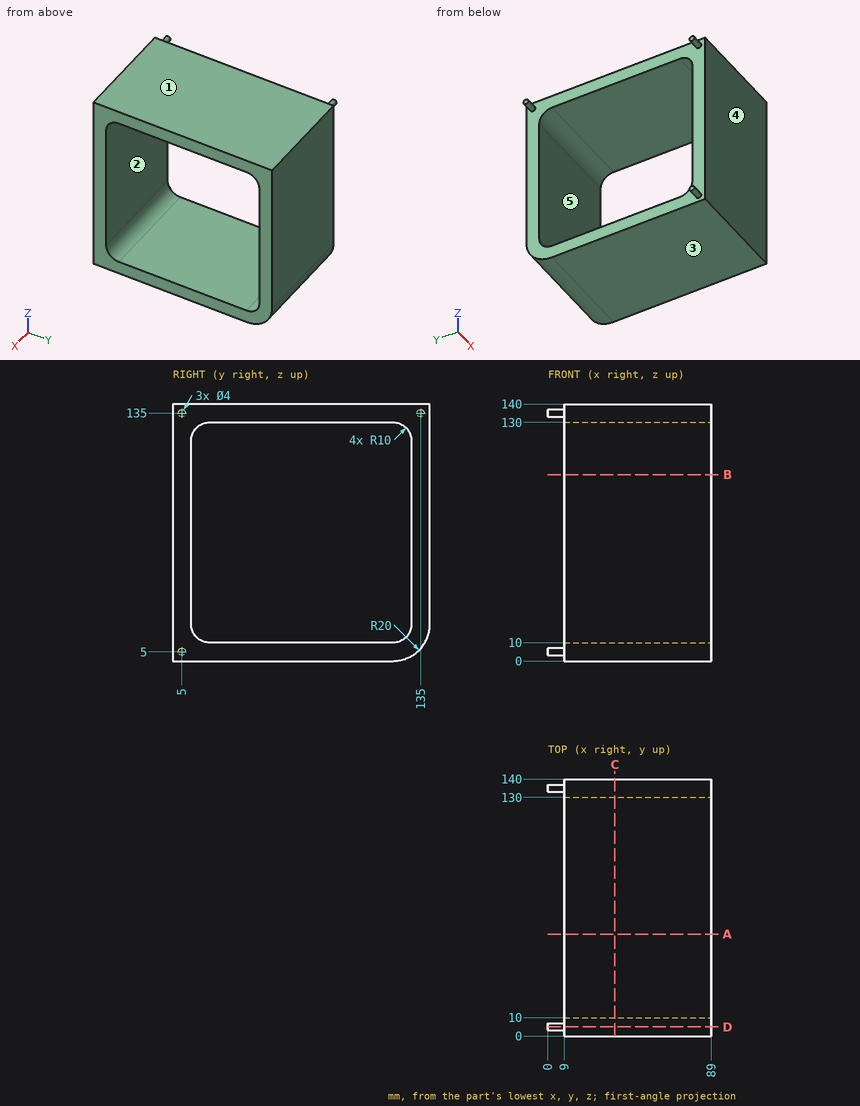
Input: dimensioned drawing with shaded views. Units: mm. Origin: part minimum x, y, z. A direction names the side the tool comes from. Coordinates: 2 decimals unless noted, no trailing zeros. Write each loop counter-clockwise with the first axis right and the second up, starting at its lowest first coordinate (ties: lowest second). Pieces come first, ordered by that corner, then holes. Notation, with made-up numbers: M -39.5,53.25 L -8.5,53.25 A16 cw -8.5,74.25 Z; hole C 41.5,84.25 d1. An arc over 180 degrees is marked long. Answer as a JSON object with one key per item and string values. Group by question number.
(1) Section A-A on y = 55.5. Output: boundary loops of the cut face in (x, z), plus the area to 3 significant figures.
(2) Mould query, pull axis Z, two halves, no side actions, for the marked faces 3, 4 and 5. Classes: pulls with the +Z half, pulls with the -Z half, needs draft (parallel to the pull), parting line crosses it, or undercut.
(3) Set-up query: the marked faces 1 and 2. Return all of +Z, -Z, +X, -X, +Y, -Y with unobstructed straight access to the full face (end or side cutting, diameter ignored); none if empty.
(4) Ray query, line 1 along Y through (x, z) = (9.5, 54); line 2 along X through (y, z) = (7, 66.5). Return the intervals inside material, ascending. Write a range as [from, to].
(5) Section D-D on y = 5. Output: boundary loops of the cut face in (x, z), plus the area to 3 significant figures.
(6) Section C-C on x = 36.5. Output: boundary loops of the cut face in (y, z), plus the area to 3 significant figures.
Result set:
{
 "1": {"outline": "M 9,0 L 89,0 L 89,10 L 9,10 Z; M 9,130 L 89,130 L 89,140 L 9,140 Z", "area": "1,600 mm2"},
 "2": {"face 3": "pulls with the -Z half", "face 4": "needs draft", "face 5": "undercut"},
 "3": {"face 1": "+Z, +X, -X, +Y, -Y", "face 2": "+X, -X"},
 "4": {"line 1": "y = [0, 10], [130, 140]", "line 2": "x = [9, 89]"},
 "5": {"outline": "M 0,3 L 9,3 L 9,0 L 89,0 L 89,140 L 9,140 L 9,137 L 0,137 L 0,133 L 9,133 L 9,7 L 0,7 Z", "area": "11,300 mm2"},
 "6": {"outline": "M 0,0 L 120,0 A20 ccw 140,20 L 140,140 L 0,140 Z; hole M 10,20 A10 ccw 20,10 L 120,10 A10 ccw 130,20 L 130,120 A10 ccw 120,130 L 20,130 A10 ccw 10,120 Z", "area": "5,200 mm2"}
}
